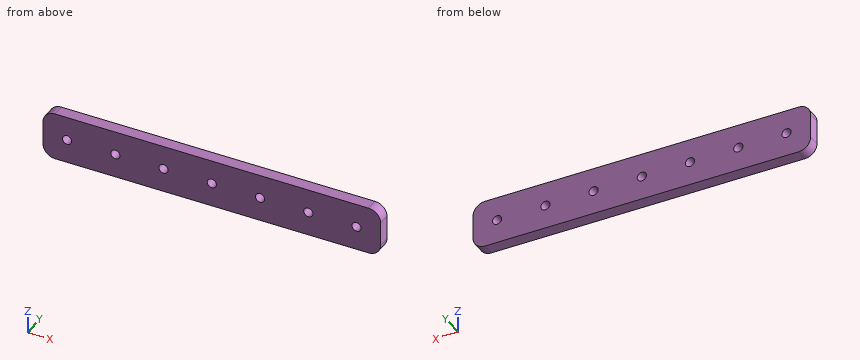
```python
from build123d import *

# Parameters (mm, degrees)
SKETCH1_W           = 177.8
SKETCH1_H           = 25.4
BOSS_EXTRUDE1_DEPTH = 6.35
SKETCH2_R           = 2.425
CUT_EXTRUDE1_DEPTH  = 6.35
FILLET1_R           = 6.35


with BuildPart() as part:
    # Sketch1 → Boss-Extrude1 (new body)
    with BuildSketch(Plane(origin=(0, 0, 0), x_dir=(1, 0, 0), z_dir=(0, 1, 0))):
        with Locations((88.9, 12.7)):
            Rectangle(SKETCH1_W, SKETCH1_H)
    extrude(amount=BOSS_EXTRUDE1_DEPTH)

    # Sketch2 → Cut-Extrude1 (cut)
    with BuildSketch(Plane(origin=(0, 6.35, 0), x_dir=(1, 0, 0), z_dir=(0, 1, 0))):
        with Locations((12.7, 12.7)):
            Circle(SKETCH2_R)
        with Locations((38.1, 12.7)):
            Circle(SKETCH2_R)
        with Locations((63.5, 12.7)):
            Circle(SKETCH2_R)
        with Locations((88.9, 12.7)):
            Circle(SKETCH2_R)
        with Locations((114.3, 12.7)):
            Circle(SKETCH2_R)
        with Locations((139.7, 12.7)):
            Circle(SKETCH2_R)
        with Locations((165.1, 12.7)):
            Circle(SKETCH2_R)
    extrude(amount=-CUT_EXTRUDE1_DEPTH, mode=Mode.SUBTRACT)

    # Fillet1
    fillet1_edges = [part.edges().sort_by_distance(p)[0] for p in [
        (0, 3.175, -25.4),
        (177.8, 3.175, -25.4),
        (177.8, 3.175, 0),
        (0, 3.175, 0),
    ]]
    fillet(fillet1_edges, radius=FILLET1_R)


solid = part.part
```
Design review of the part built by this model. Coordinates are the model's own, in mm. Give positions to 0.01 mm unless a question says otherwise; leave off trailing zeros. Loops run counter-clockwise (first coordinate to the right, second up) from the corner with the lowest first, then second, coordinate; pieces in that order, holes last. Notation, with made-up numbers: (21.5, 39) -> (45.5, 39) arc R21 ccw to (45.5, 70) -> close; hole circle Ø7 at (46, 86). An arc over 180 degrees is marked (long way). One line per item, written item: value.
Q1. We need section A-A on y = 5. Give the boundary of the cut face in (x, z) (3 decimals).
Numbers:
outline: (0, -19.05) arc R6.35 ccw to (6.35, -25.4) -> (171.45, -25.4) arc R6.35 ccw to (177.8, -19.05) -> (177.8, -6.35) arc R6.35 ccw to (171.45, 0) -> (6.35, 0) arc R6.35 ccw to (0, -6.35) -> close; hole circle Ø4.85 at (12.7, -12.7); hole circle Ø4.85 at (38.1, -12.7); hole circle Ø4.85 at (63.5, -12.7); hole circle Ø4.85 at (88.9, -12.7); hole circle Ø4.85 at (114.3, -12.7); hole circle Ø4.85 at (139.7, -12.7); hole circle Ø4.85 at (165.1, -12.7)
Q2. We need section B-B on x = 165.1. Give the boundary of the cut face in (y, z) (3 decimals), and give its area (3 significant figures).
Numbers:
outline: (0, -25.4) -> (6.35, -25.4) -> (6.35, -15.125) -> (0, -15.125) -> close; (0, -10.275) -> (6.35, -10.275) -> (6.35, 0) -> (0, 0) -> close
area: 130 mm^2
Q3. We need section C-C on z = -12.7. Give the number of separate pieces and of enclosed holes in the cut face, and give its area (3 significant figures).
Numbers:
separate pieces: 8
enclosed holes: 0
area: 913 mm^2
Q4. For L1, parallel to Z at x = 88.9, y = 4.75 (3 decimals); L2, parallel to X at y = 3.5, z = -19.5; L3, parallel to X at y = 4.5, z = -23, list the stretches that pass through material, from the lowest coordinate up.
Numbers:
L1: z = -25.4 to -15.125, -10.275 to 0
L2: x = 0.02 to 177.78
L3: x = 1.38 to 176.42
